from build123d import *

# Parameters (mm, degrees)
RESSALTO_EXTRUS_O1_DEPTH   = 20
ESBO_O2_R                  = 2
CORTE_EXTRUS_O1_DEPTH      = 12
CORTE_EXTRUS_O1_DEPTH_BACK = 16


with BuildPart() as part:
    # Esboço1 → Ressalto-extrusão1 (new body)
    with BuildSketch(Plane.XY):
        with BuildLine():
            Line((3.196343382, -1.5), (3.583399622, -1.5))
            Line((3.583399622, -1.5), (5.483399622, -1.5))
            Line((5.483399622, -1.5), (3.796667791, 0.712536536))
            ThreePointArc((3.796667791, 0.712536536), (3.093538771, 1.292355025), (2.206147389, 1.5))
            Line((2.206147389, 1.5), (-2.51439317, 1.5))
            ThreePointArc((-2.51439317, 1.5), (-3.488374138, 1.24681455), (-4.215757297, 0.551361073))
            Line((-4.215757297, 0.551361073), (-5.483399622, -1.5))
            Line((-5.483399622, -1.5), (-4.016600378, -1.5))
            Line((-4.016600378, -1.5), (-4.016600378, -4.5))
            Line((-4.016600378, -4.5), (1.196343382, -4.5))
            Line((1.196343382, -4.5), (1.196343382, -7.5))
            Line((1.196343382, -7.5), (-4.016600378, -7.5))
            Line((-4.016600378, -7.5), (-4.016600378, -10.5))
            Line((-4.016600378, -10.5), (3.196343382, -10.5))
            Line((3.196343382, -10.5), (3.196343382, -7.5))
            Line((3.196343382, -7.5), (3.196343382, -4.5))
            Line((3.196343382, -4.5), (3.196343382, -1.5))
        make_face()
    extrude(amount=RESSALTO_EXTRUS_O1_DEPTH)

    # Esboço2 → Corte-extrusão1 (cut, two sides)
    with BuildSketch(Plane(origin=(0, 0, 0), x_dir=(1, 0, 0), z_dir=(0, 1, 0))) as corte_extrus_o1_sk:
        with Locations((-0.15412289, -3.574880423)):
            Circle(ESBO_O2_R)
        with Locations((-0.15412289, -10.26404601)):
            Circle(ESBO_O2_R)
        with Locations((-0.15412289, -16.953211597)):
            Circle(ESBO_O2_R)
    extrude(amount=CORTE_EXTRUS_O1_DEPTH, mode=Mode.SUBTRACT)
    extrude(corte_extrus_o1_sk.sketch, amount=-CORTE_EXTRUS_O1_DEPTH_BACK, mode=Mode.SUBTRACT)


solid = part.part
Geometry: final body of the model. Coordinates: model frame, mm. A direction names the side the tool comes from. Give positions to 0.01 mm unless a question says otherwise; leave off trailing zeros. Loops run counter-clockwise (first coordinate to the right, second up) from the corner with the lowest first, then second, coordinate; pieces in that order, holes last. Notation, with made-up numbers: (73, 20.5) - (126, 20.5) arc R23 cw to (126, 43.5) - close; hole circle Ø11 at (42, 76.25). An arc over 180 degrees is marked (long way). One line per question, with ' | ' between items. Start each with the question number.
(1) Pull-direction query (Y, two-part tool) for faces 4 (the flat face through (-5, -1.5, 10)), 5 (the cylindrical face through (1.754, -4.416, 2.974)), 6 (the flat face through (-3, -4.5, 10)), 7 (the flat face through (0, 1.5, 8)); classes: released by +Y, released by -Y, zero draft, split by the parting line, or undercut.
(2) Ray query, line 1 (Z direction, x = 0, y = 0.25); line 2 (Y direction, x = -2.5, z = 9); line 3 (Z direction, x = 0.25, y = -1.5). Return the intervals inside material, ascending. Write a range as from..to.
(3) Contact query for flat-ended pins moving along their axis: pin 1 (1.2 mm diameter, centred on x = -5, z = 14, fed in from -Y); pin 2 (0.9 mm diameter, centred on y = -5.5, z = 13, fed in from -X); pin 3 (1.5 mm diameter, centred on y = -3, z = 13, fed in from -X). Output: stop coordinate, or through.
(4) Reachability of faces 1 (the flat face through (-4.017, -9, 10)), 2 (the flat face through (1.196, -6, 14)), 3 (the flat face through (3.196, -6, 10)) from +Z, -Z, +X, -X, +Y, -Y: full face, straight path, thin tool, end or side. Return the list, or none.
(5) Section query A-A on x = -3.5. Return loops of the section in (y, z).
(6) Section query C-C on y = -5.5. Return loops of the section in (x, z).
(7) Section query B-B on z = 7. Return loops of the section in (x, y), then the cut area to 3 significant figures.
(8) Section query D-D on y = -0.5. Return loops of the section in (x, z), then the cut area to 3 significant figures.
The answers:
1) face 4: released by -Y | face 5: zero draft | face 6: undercut | face 7: released by +Y
2) line 1: 0..1.58, 5.57..8.27, 12.26..14.96, 18.95..20 | line 2: -10.5..-7.5, -4.5..1.5 | line 3: 0..1.62, 5.53..8.31, 12.22..14.99, 18.91..20
3) pin 1: y = -1.5 | pin 2: x = 1.2 | pin 3: x = -4.02
4) face 1: +Z, -Z, -X, -Y | face 2: +Z, -Z, -X | face 3: +Z, -Z, +X, -Y
5) outline: (-10.5, 0) - (-7.5, 0) - (-7.5, 20) - (-10.5, 20) - close; (-4.5, 0) - (1.24, 0) - (1.24, 20) - (-4.5, 20) - close
6) outline: (1.2, 0) - (3.2, 0) - (3.2, 20) - (1.2, 20) - (1.2, 18.43) arc R2 cw to (1.2, 15.48) - (1.2, 11.74) arc R2 cw to (1.2, 8.79) - (1.2, 5.05) arc R2 cw to (1.2, 2.1) - close
7) outline: (-5.48, -1.5) - (-4.02, -1.5) - (-4.02, -4.5) - (1.2, -4.5) - (1.2, -7.5) - (-4.02, -7.5) - (-4.02, -10.5) - (3.2, -10.5) - (3.2, -1.5) - (5.48, -1.5) - (3.8, 0.71) arc R2 ccw to (2.21, 1.5) - (-2.51, 1.5) arc R2 ccw to (-4.22, 0.55) - close | area: 75.6 mm2
8) outline: (-4.87, 0) - (4.72, 0) - (4.72, 20) - (-4.87, 20) - close; hole circle Ø4 at (-0.15, 3.57); hole circle Ø4 at (-0.15, 10.26); hole circle Ø4 at (-0.15, 16.95) | area: 154 mm2
